```python
from build123d import *


with BuildPart() as part:
    # Sketch1 → Revolve1 (revolve)
    with BuildSketch(Plane.XY):
        with BuildLine():
            Line((0, -17.935), (0, -30))
            Line((0, -30), (10, -30))
            Line((10, -30), (12.580192505, -20))
            Line((12.580192505, -20), (22.320508076, -20))
            Line((22.320508076, -20), (25, -30))
            Line((25, -30), (35, -30))
            Line((35, -30), (35, -20))
            Line((35, -20), (44.5, -20))
            ThreePointArc((44.5, -20), (44.853553391, -19.853553391), (45, -19.5))
            Line((45, -19.5), (45, -7.935))
            Line((45, -7.935), (2.5, -7.935))
            Line((2.5, -7.935), (0, -17.935))
        make_face()
    revolve(axis=Axis((0, 0, 0), (1, 0, 0)))


solid = part.part
```
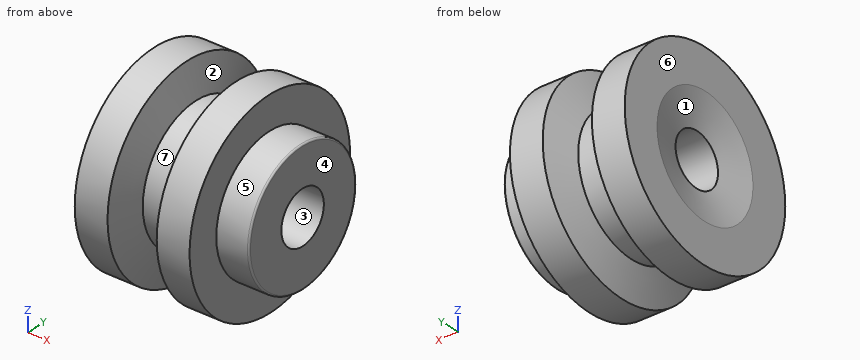
Read the model definition and answer for the solid it produces. Units are mm, in the model's axes. Face numbers are marked on the shaded views. A direction names the side the tool comes from. Coordinates: 2 decimals unless noted, no trailing zeros. Order: outer loops, then holes, each group sorted by start corner. A loop starts at its lowest first (then second) coordinate and runs counter-clockwise, first axis right, second up. Notation, with made-up numbers: (82, -13) - (134, -13) arc R19 cw to (134, 24) - close; hole circle Ø7 at (77.5, 54.25). An arc over 180 degrees is marked (long way). Answer as a JSON object with one key per item and string values. Group by question number.
Item 1: Section D-D (x = 16) is taken. Give the vertices of the cut face in (y, z) (3 decimals).
Item 2: Consider probe 1 along Y at (x, z) = (19, 0) (3 decimals); probe 2 along Z at (x, y) = (27, 0) (3 decimals). Determine where each line is inside the solid, lowest interval first. Write a range as from..to.
Item 3: Section A-A (y = 0) is taken. Give the vertices of the cut face in (x, z) (1 decimal).
Item 4: Flat-ended cylindrical pins translate along their axes: P1, Ø10, axis at y = -18.5, z = 3.5, coming from the -X side; P2, Ø3, axis at x = 29, y = -5, coming from the -Z side; P3, Ø2, axis at x = 33, y = -15.5, coming from the +Z side; P4, Ø8, axis at x = 23.5, z = 20.5, coming from the +Y side. Find the tip coordinate at first contact, or state that the pin passes through.
Item 5: A tool of negligible diameter and unlimited length cuts with its end or side. For the marked faces 5, 6 and 7, from which of +Z, -Z, +X, -X, +Y, -Y can it reach the whole face along a straight path? Write none if from no direction.
Item 6: Section C-C (x = 6.5) is taken. Give the vertices of the cut face in (y, z) (3 decimals), plus the area to 3 significant figures.
Item 7: The mould has two halves that part along Z. Classify the marked faces 1, 2, 3 and 4: +Z half, -Z half, draft (parallel to the pull), parting line (faces both ways), or undercut.
Results are:
{
 "1": {"outline": "circle Ø40 at (0, 0); hole circle Ø15.87 at (0, 0)"},
 "2": {"probe 1": "y = -20..-7.935, 7.935..20", "probe 2": "z = -30..-7.935, 7.935..30"},
 "3": {"outline": "(0, -30) - (10, -30) - (12.6, -20) - (22.3, -20) - (25, -30) - (35, -30) - (35, -20) - (44.5, -20) arc R0.5 ccw to (45, -19.5) - (45, -7.9) - (2.5, -7.9) - (0, -17.9) - close; (0, 17.9) - (2.5, 7.9) - (45, 7.9) - (45, 19.5) arc R0.5 ccw to (44.5, 20) - (35, 20) - (35, 30) - (25, 30) - (22.3, 20) - (12.6, 20) - (10, 30) - (0, 30) - close"},
 "4": {"P1": "stops at x = 0", "P2": "stops at z = -29.8", "P3": "stops at z = 26.26", "P4": "stops at y = 24.86"},
 "5": {"face 5": "+X", "face 6": "+Z, -Z, -X, +Y, -Y", "face 7": "none"},
 "6": {"outline": "circle Ø60 at (0, 0); hole circle Ø15.87 at (0, 0)", "area": "2,630 mm^2"},
 "7": {"face 1": "undercut", "face 2": "parting line", "face 3": "undercut", "face 4": "draft"}
}
